Can you work these out from the model? Positions are in its coordinate system, mm. Face numbers are marked on the shaded views. A direction names the side the tool comes from. Give positions to 0.01 mm unless a question says otherwise; leave off trailing zeros. Order: outer loops, then holes, each group sorted by start corner. A loop starts at its lowest first (then second) coordinate and runs counter-clockwise, first axis right, second up. Notation, with made-up numbers: (61.25, 77) - (111.25, 77) arc R23 ccw to (111.25, 116) - close; hole circle Ø4 at (58.25, 16.25). An arc over 180 degrees is marked (long way). One line per question, with ' | ' between items.
```python
from build123d import *

# Parameters (mm, degrees)
SKETCH1_W           = 17
SKETCH1_H           = 29.7
BOSS_EXTRUDE1_DEPTH = 22
SKETCH2_R           = 2
CUT_EXTRUDE1_DEPTH  = 30.7
SKETCH3_R           = 4
CUT_EXTRUDE2_DEPTH  = 27.7
CUT_EXTRUDE4_START  = -2
SKETCH4_W           = 13
SKETCH4_H           = 18
CUT_EXTRUDE4_DEPTH  = 25.7


with BuildPart() as part:
    # Sketch1 → Boss-Extrude1 (new body)
    with BuildSketch(Plane.XY):
        with Locations((8.5, 14.85)):
            Rectangle(SKETCH1_W, SKETCH1_H)
    extrude(amount=BOSS_EXTRUDE1_DEPTH)

    # Sketch2 → Cut-Extrude1 (cut, through all)
    with BuildSketch(Plane(origin=(0, 29.7, 0), x_dir=(1, 0, 0), z_dir=(0, 1, 0))):
        with Locations((8.5, -11)):
            Circle(SKETCH2_R)
    extrude(amount=-CUT_EXTRUDE1_DEPTH, mode=Mode.SUBTRACT)

    # Sketch3 → Cut-Extrude2 (cut)
    with BuildSketch(Plane.XZ):
        with Locations((8.5, 11)):
            Circle(SKETCH3_R)
    extrude(amount=-CUT_EXTRUDE2_DEPTH, mode=Mode.SUBTRACT)

    # Sketch4 → Cut-Extrude4 (cut)
    with BuildSketch(Plane.XZ.offset(CUT_EXTRUDE4_START)):
        with Locations((8.5, 11)):
            Rectangle(SKETCH4_W, SKETCH4_H)
    extrude(amount=-CUT_EXTRUDE4_DEPTH, mode=Mode.SUBTRACT)


solid = part.part
```
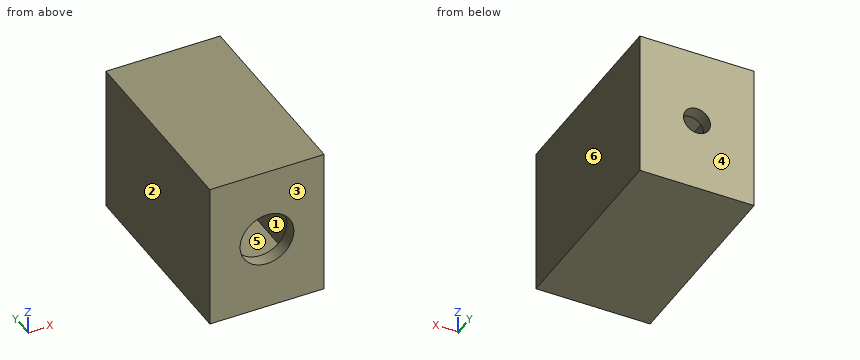
(1) Imagine slicing it at D-D (z = 11). List the corners of the cut face in (x, y) for me.
Answer below:
outline: (0, 0) - (4.5, 0) - (4.5, 2) - (2, 2) - (2, 27.7) - (6.5, 27.7) - (6.5, 29.7) - (0, 29.7) - close; (10.5, 27.7) - (15, 27.7) - (15, 2) - (12.5, 2) - (12.5, 0) - (17, 0) - (17, 29.7) - (10.5, 29.7) - close
(2) On a 3-axis mill with a long thin cutter (end or side, diameter ignored), from which of +Z, -Z, +X, -X, +Y, -Y can I reach the whole of each face in a straight line? I mean the marked faces 1 and 2. Say none if no direction works.
Answer below:
face 1: none | face 2: +Z, -Z, -X, +Y, -Y
(3) Will this pin go through, and if not, where does the flat tip stop? pin 1 (2.5 mm diameter, centred on x = 8.5, z = 11, fed in from -Y).
Answer below:
pin 1: through
(4) If we mould it in two halves opening along Y, with no side actions, what happens to the marked faces 3, 4, 5 and 6? For each: released by +Y, released by -Y, zero draft, split by the parting line, or undercut.
Answer below:
face 3: released by -Y | face 4: released by +Y | face 5: undercut | face 6: zero draft
(5) If I drill on line 1 (Z direction, x = 10.25, y = 10); line 2 (X direction, y = 7.75, z = 13); line 3 (Z direction, x = 8.5, y = 28.45), over which ranges is the centre line in solid material (lowest first)?
Answer below:
line 1: 0 to 2, 20 to 22 | line 2: 0 to 2, 15 to 17 | line 3: 0 to 9, 13 to 22
(6) Imagine slicing it at C-C (x = 8.5). List the corners of the cut face in (y, z) for me.
Answer below:
outline: (0, 0) - (29.7, 0) - (29.7, 9) - (27.7, 9) - (27.7, 2) - (2, 2) - (2, 7) - (0, 7) - close; (0, 15) - (2, 15) - (2, 20) - (27.7, 20) - (27.7, 13) - (29.7, 13) - (29.7, 22) - (0, 22) - close
(7) Imagine slicing it at B-B (y = 14.25). List the corners of the cut face in (x, z) for me, and give its area (3 significant figures).
Answer below:
outline: (0, 0) - (17, 0) - (17, 22) - (0, 22) - close; hole (2, 2) - (15, 2) - (15, 20) - (2, 20) - close | area: 140 mm^2
(8) Imagine slicing it at A-A (z = 4). List the corners of the cut face in (x, y) for me.
Answer below:
outline: (0, 0) - (17, 0) - (17, 29.7) - (0, 29.7) - close; hole (2, 2) - (15, 2) - (15, 27.7) - (2, 27.7) - close
